The figure shows three views and two pictorial views of one solid part (mm, origin at its lowest corner). Answer the questions. A direction names the side the tool comes from. Round coordinates to 2 decimals unless told otherwise and drop trailing zeros. Write each loop counter-clockwise with the first axis right and the second up, starting at its lowest first coordinate (ties: lowest second). Pieces come first, ordered by that corner, then holes.
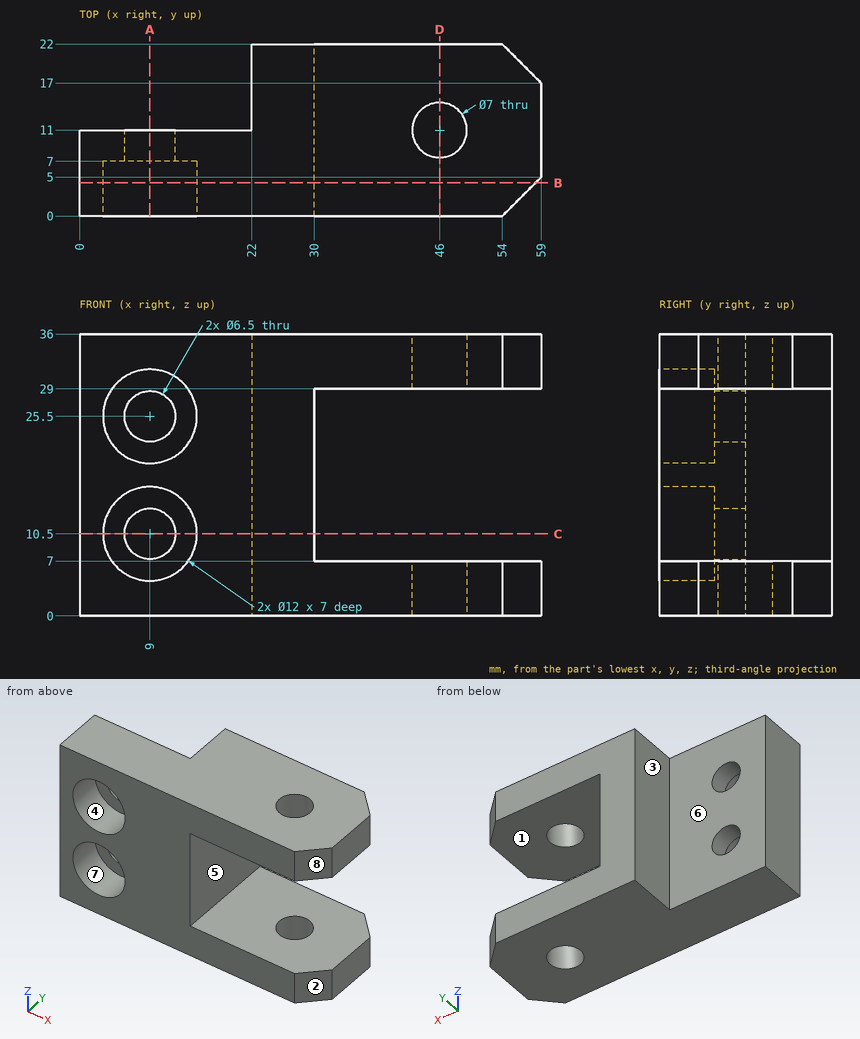
Q1. Flat-ended cylindrical pins translate along their axes: pin 1 Ø8.5 at (x, z) = (9, 25.5) entering from -Y; pin 2 Ø6.5 at (y, z) = (14.5, 17.5) entering from +X; pin 3 Ø17.5 at (x, z) = (10.5, 14.5) entering from +Y. Find the tip coordinate at first contact, or state that the pin passes through.
Verdict:
pin 1: stops at y = 7
pin 2: stops at x = 30
pin 3: stops at y = 11
Q2. Section D-D (x = 46) is taken. Determine the outline of the cut face in (y, z).
Verdict:
outline: (0, 0) - (7.5, 0) - (7.5, 7) - (0, 7) - close; (0, 29) - (7.5, 29) - (7.5, 36) - (0, 36) - close; (14.5, 0) - (22, 0) - (22, 7) - (14.5, 7) - close; (14.5, 29) - (22, 29) - (22, 36) - (14.5, 36) - close
Q3. Section C-C (z = 10.5) is taken. Determine the outline of the cut face in (x, y), then the cut area to 3 significant figures.
Verdict:
outline: (0, 0) - (3, 0) - (3, 7) - (5.75, 7) - (5.75, 11) - (0, 11) - close; (12.25, 7) - (15, 7) - (15, 0) - (30, 0) - (30, 22) - (22, 22) - (22, 11) - (12.25, 11) - close
area: 308 mm2
Q4. Section B-B (y = 4.25) is taken. Determine the outline of the cut face in (x, z), then the cut area to 3 significant figures.
Verdict:
outline: (0, 0) - (58.25, 0) - (58.25, 7) - (30, 7) - (30, 29) - (58.25, 29) - (58.25, 36) - (0, 36) - close; hole circle Ø12 at (9, 10.5); hole circle Ø12 at (9, 25.5)
area: 1,250 mm2
Q5. Determine the mould class of the marked faces 1, 2, 3 and 4 for opening direction X: pulls with the +X half, pulls with the -X half, needs draft (parallel to the pull), parting line crosses it, or undercut.
Verdict:
face 1: needs draft
face 2: pulls with the +X half
face 3: pulls with the -X half
face 4: undercut
Q6. Straight lines are drawn through the part: probe 1 along Z at (x, y) = (9, 4); probe 2 along Z at (x, y) = (51.5, 6.75); probe 3 along X at (y, z) = (16.25, 27). For each, find the intervals that lie inside material, in ascending order.
Verdict:
probe 1: z = 0 to 4.5, 16.5 to 19.5, 31.5 to 36
probe 2: z = 0 to 7, 29 to 36
probe 3: x = 22 to 30
Q7. Which of the six approach directions +Z, -Z, +X, -X, +Y, -Y give full straight-line access (tool end or side, diameter ignored) to the marked faces 5, 6, 7 and 8?
Verdict:
face 5: +X, +Y, -Y
face 6: +Z, -Z, -X, +Y
face 7: -Y
face 8: +Z, -Z, +X, -Y
Q8. Section A-A (x = 9) is taken. Determine the outline of the cut face in (y, z), then the cut area to 3 significant figures.
Verdict:
outline: (0, 0) - (11, 0) - (11, 7.25) - (7, 7.25) - (7, 4.5) - (0, 4.5) - close; (0, 16.5) - (7, 16.5) - (7, 13.75) - (11, 13.75) - (11, 22.25) - (7, 22.25) - (7, 19.5) - (0, 19.5) - close; (0, 31.5) - (7, 31.5) - (7, 28.75) - (11, 28.75) - (11, 36) - (0, 36) - close
area: 176 mm2
